from build123d import *

# Parameters (mm, degrees)
SKETCH063_R     = 1.75
PAD039_DEPTH    = 8
SKETCH064_R     = 4.9
POCKET025_DEPTH = 38
SKETCH065_R     = 1.6
POCKET026_DEPTH = 10


with BuildPart() as part:
    # Sketch063 → Pad039 (new body)
    with BuildSketch(Plane.XZ):
        Polygon((-15, -16), (15, -16), (33.595724, -10.458334), (33.595724, 0), (15, 16), (-15, 16), align=None)
        with Locations((-10, 0)):
            Circle(SKETCH063_R, mode=Mode.SUBTRACT)
        with Locations((10, 4)):
            Circle(SKETCH063_R, mode=Mode.SUBTRACT)
        with Locations((10, -4)):
            Circle(SKETCH063_R, mode=Mode.SUBTRACT)
    extrude(amount=PAD039_DEPTH)

    # Sketch064 (on Face3 of Pad039) → Pocket025 (cut)
    with BuildSketch(Plane(origin=(0, 0, -16), x_dir=(1, 0, 0), z_dir=(0, 0, -1))):
        Circle(SKETCH064_R)
    extrude(amount=-POCKET025_DEPTH, mode=Mode.SUBTRACT)

    # Sketch065 (on Face2 of Pocket025) → Pocket026 (cut)
    with BuildSketch(Plane(origin=(0, 0, 0), x_dir=(1, 0, 0), z_dir=(0, 1, 0))):
        with Locations((26.9, 5)):
            Circle(SKETCH065_R)
        with Locations((-10, 10)):
            Circle(SKETCH065_R)
        with Locations((10, 10)):
            Circle(SKETCH065_R)
        with Locations((10, -10)):
            Circle(SKETCH065_R)
        with Locations((-10, -10)):
            Circle(SKETCH065_R)
    extrude(amount=-POCKET026_DEPTH, mode=Mode.SUBTRACT)


with BuildPart() as part_1:
    # Body011 placement: moved
    add(part.part.moved(Location((-1.1, -53.7, 39.5))))


solid = part_1.part
Could you check a few things on this model? Use its own coordinates, in mm. Coordinates: 2 decimals unless noted, no trailing zeros. Order: outer loops, then holes, each group sorted by start corner. A loop starts at its lowest first (then second) coordinate and runs counter-clockwise, first axis right, second up. Notation, with made-up numbers: (-31.75, -22.75) - (23.25, -22.75) arc R18 ccw to (23.25, -17.75) - close; hole circle Ø9 at (31.25, -3). An arc over 180 degrees is marked (long way). Answer in a Markdown table with one row per item. Add a question column.
(1) I need wall thicknesses on L1, parallel to X at y = -60, z = 29.5; L2, parallel to Z at x = 8.9, y = -56; L3, parallel to Z at x = -11.1, y = -59.5. Which ranges of each line are inside material? Lowest first, please.
(2) If we section it at B-B, the plane y = -55: State how many separate pieces and enclosed holes the cut face has, then the cut area to 3 significant figures.
(3) Will these pins go through, and if not, where does the flat tip stop? pin 1 (4 mm diameter, centred on y = -57, z = 50.5, fed in from +X); pin 2 (2 mm diameter, centred on y = -60, z = 52, fed in from +X).
(4) If we section it at C-C, the plane x = 8.9: Please give me the cut outline in (y, z).
(5) If we section it at D-D, the plane z = 30: Please give me the cut outline in (x, y).
(6) If we section it at A-A, the plane x = -11.1: Please give me the cut outline in (y, z).
(7) If we mould it in two halves opening along Z, with no side actions, what happens to faces 1 (the face through (-1, -58.6, 39.3)), 2 (the face through (-1, -59, 23.5)), 3 (the face through (8.692, -57.644, 27.914))? For each: released by +Z, released by -Z, zero draft, split by the parting line, or undercut.
Results are:
| question | item | result |
|---|---|---|
| 1 | L1 | x = -16.1 to -12.7, -9.5 to 7.3, 10.5 to 32.5 |
| 1 | L2 | z = 23.5 to 27.9, 31.1 to 33.75, 37.25 to 41.75, 45.25 to 47.9, 51.1 to 55.5 |
| 1 | L3 | z = 23.5 to 27.9, 31.1 to 37.75, 41.25 to 47.9, 51.1 to 55.5 |
| 2 | separate pieces | 2 |
| 2 | enclosed holes | 8 |
| 2 | area | 983 mm2 |
| 3 | pin 1 | stops at x = 22.04 |
| 3 | pin 2 | stops at x = 19.13 |
| 4 | outline | (-61.7, 23.5) - (-53.7, 23.5) - (-53.7, 27.9) - (-61.7, 27.9) - close; (-61.7, 31.1) - (-53.7, 31.1) - (-53.7, 33.75) - (-61.7, 33.75) - close; (-61.7, 37.25) - (-53.7, 37.25) - (-53.7, 41.75) - (-61.7, 41.75) - close; (-61.7, 45.25) - (-53.7, 45.25) - (-53.7, 47.9) - (-61.7, 47.9) - close; (-61.7, 51.1) - (-53.7, 51.1) - (-53.7, 55.5) - (-61.7, 55.5) - close |
| 5 | outline | (-16.1, -61.7) - (-12.62, -61.7) - (-12.62, -53.7) - (-16.1, -53.7) - close; (-9.58, -61.7) - (7.38, -61.7) - (7.38, -53.7) - (3.8, -53.7) arc R4.9 cw to (-6, -53.7) - (-9.58, -53.7) - close; (10.42, -61.7) - (32.5, -61.7) - (32.5, -53.7) - (10.42, -53.7) - close |
| 6 | outline | (-61.7, 23.5) - (-53.7, 23.5) - (-53.7, 27.9) - (-61.7, 27.9) - close; (-61.7, 31.1) - (-53.7, 31.1) - (-53.7, 37.75) - (-61.7, 37.75) - close; (-61.7, 41.25) - (-53.7, 41.25) - (-53.7, 47.9) - (-61.7, 47.9) - close; (-61.7, 51.1) - (-53.7, 51.1) - (-53.7, 55.5) - (-61.7, 55.5) - close |
| 7 | face 1 | zero draft |
| 7 | face 2 | released by -Z |
| 7 | face 3 | undercut |
